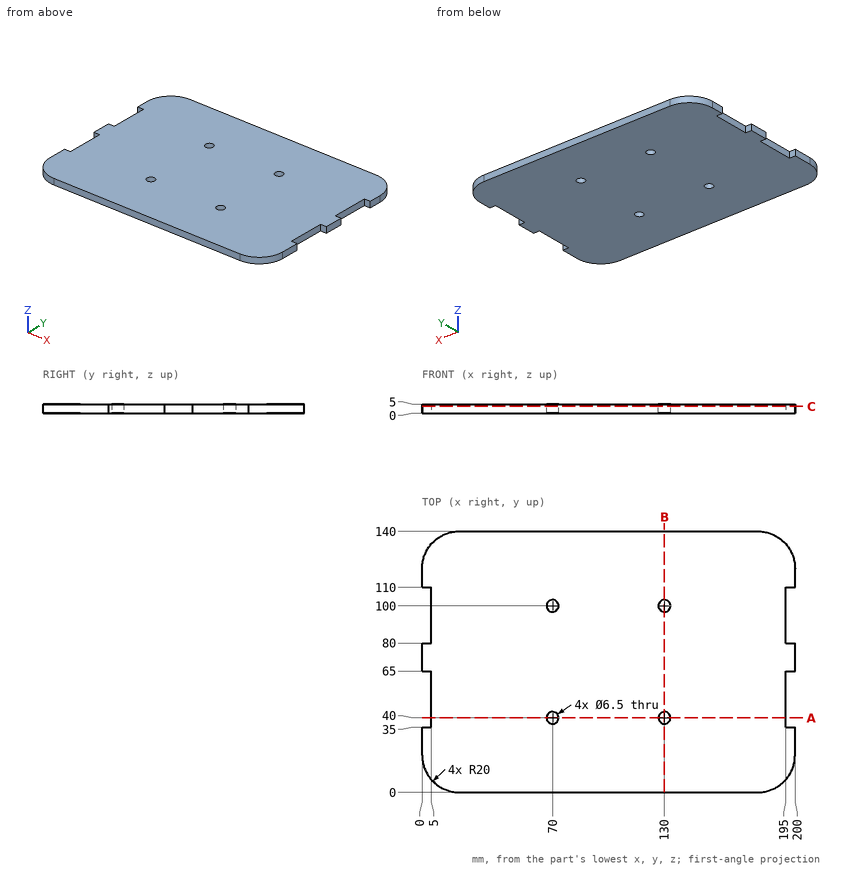
Job drawing, mm, ordinate dimensions from the low corner. One solid piece. Give positions to 0.01 mm unless a question says otherwise; leave off trailing zeros. Write each loop counter-clockwise with the first axis right and the second up, starting at its lowest first coordinate (ties: lowest second). Pieces come first, ordered by that corner, then holes. Notation, with made-up numbers: (79, 0) -> (85, 0) arc R23 cw to (85, 37) -> close; hole circle Ø2 at (80.5, -25.5). An arc over 180 degrees is marked (long way). Return JSON: item names as keys, results as strings.
Item 1: Band-saw the part on B-B (x = 130). List the corners of the cut face in (y, z), then the cut area to 3 significant figures.
Answer below:
{"outline": "(0, 0) -> (36.75, 0) -> (36.75, 5) -> (0, 5) -> close; (43.25, 0) -> (96.75, 0) -> (96.75, 5) -> (43.25, 5) -> close; (103.25, 0) -> (140, 0) -> (140, 5) -> (103.25, 5) -> close", "area": "635 mm2"}
Item 2: Drill centre lines: probe 1 along Y at (x, z) = (70, 3.75); probe 2 along X at (y, z) = (102.5, 4.7); probe 3 along X at (y, z) = (57, 1.45). Where is each one in solid material? Low to high.
Answer below:
{"probe 1": "y = 0 to 36.75, 43.25 to 96.75, 103.25 to 140", "probe 2": "x = 5 to 67.92, 72.08 to 127.92, 132.08 to 195", "probe 3": "x = 5 to 195"}
Item 3: Band-saw the part on C-C (z = 3.7). List the corners of the cut face in (x, y), then the cut area to 3 significant figures.
Answer below:
{"outline": "(0, 20) arc R20 ccw to (20, 0) -> (180, 0) arc R20 ccw to (200, 20) -> (200, 35) -> (195, 35) -> (195, 65) -> (200, 65) -> (200, 80) -> (195, 80) -> (195, 110) -> (200, 110) -> (200, 120) arc R20 ccw to (180, 140) -> (20, 140) arc R20 ccw to (0, 120) -> (0, 110) -> (5, 110) -> (5, 80) -> (0, 80) -> (0, 65) -> (5, 65) -> (5, 35) -> (0, 35) -> close; hole circle Ø6.5 at (70, 40); hole circle Ø6.5 at (70, 100); hole circle Ø6.5 at (130, 40); hole circle Ø6.5 at (130, 100)", "area": "26,900 mm2"}
Item 4: Band-saw the part on A-A (y = 40). List the corners of the cut face in (x, z).
Answer below:
{"outline": "(5, 0) -> (66.75, 0) -> (66.75, 5) -> (5, 5) -> close; (73.25, 0) -> (126.75, 0) -> (126.75, 5) -> (73.25, 5) -> close; (133.25, 0) -> (195, 0) -> (195, 5) -> (133.25, 5) -> close"}
Item 5: Drop flat-ended pins along their axis: pin 1 (2.5 mm diameter, centred on y = 101, z = 2.5, fed in from +X); pin 2 (2.5 mm diameter, centred on x = 196.5, z = 2.5, fed in from -Y); pin 3 (12 mm diameter, centred on x = 166, y = 18.5, fed in from -Z); pin 4 (2.5 mm diameter, centred on x = 1.5, z = 3.5, fed in from -Y). Give the stop position or say it passes through.
Answer below:
{"pin 1": "stops at x = 195", "pin 2": "stops at y = 7.06", "pin 3": "stops at z = 0", "pin 4": "stops at y = 9.88"}
